```python
from build123d import *

# Parameters (mm, degrees)
SKETCH1_W           = 76.2
SKETCH1_H           = 50.8
SKETCH1_R           = 2.38125
BOSS_EXTRUDE1_DEPTH = 3.0988
FILLET1_R           = 3.175
SKETCH2_W           = 63.5
SKETCH2_H           = 38.1
CUT_EXTRUDE1_DEPTH  = 46.895234627
FILLET3_R           = 3.175


with BuildPart() as part:
    # Sketch1 → Boss-Extrude1 (new body)
    with BuildSketch(Plane.XY):
        Rectangle(SKETCH1_W, SKETCH1_H)
        with Locations((-25.4, 12.7)):
            Circle(SKETCH1_R, mode=Mode.SUBTRACT)
        with Locations((0, 12.7)):
            Circle(SKETCH1_R, mode=Mode.SUBTRACT)
        with Locations((25.4, 12.7)):
            Circle(SKETCH1_R, mode=Mode.SUBTRACT)
        with Locations(Location((25.4, -12.7, 0), (0, 0, 180))):
            Circle(SKETCH1_R, mode=Mode.SUBTRACT)
        with Locations(Location((0, -12.7, 0), (0, 0, 180))):
            Circle(SKETCH1_R, mode=Mode.SUBTRACT)
        with Locations(Location((-25.4, -12.7, 0), (0, 0, 180))):
            Circle(SKETCH1_R, mode=Mode.SUBTRACT)
    extrude(amount=BOSS_EXTRUDE1_DEPTH)

    # Fillet1
    fillet1_edges = [part.edges().sort_by_distance(p)[0] for p in [
        (-38.1, 25.4, 1.5494),
        (38.1, 25.4, 1.5494),
        (38.1, -25.4, 1.5494),
        (-38.1, -25.4, 1.5494),
    ]]
    fillet(fillet1_edges, radius=FILLET1_R)

    # Sketch2 → Cut-Extrude1 (cut, through all)
    with BuildSketch(Plane.XY.offset(3.0988)):
        with BuildLine():
            Line((38.1, -22.225), (38.1, 22.225))
            ThreePointArc((38.1, 22.225), (37.17006403, 24.47006403), (34.925, 25.4))
            Line((34.925, 25.4), (-34.925, 25.4))
            ThreePointArc((-34.925, 25.4), (-37.17006403, 24.47006403), (-38.1, 22.225))
            Line((-38.1, 22.225), (-38.1, -22.225))
            ThreePointArc((-38.1, -22.225), (-37.17006403, -24.47006403), (-34.925, -25.4))
            Line((-34.925, -25.4), (34.925, -25.4))
            ThreePointArc((34.925, -25.4), (37.17006403, -24.47006403), (38.1, -22.225))
        make_face()
        Rectangle(SKETCH2_W, SKETCH2_H, mode=Mode.SUBTRACT)
    extrude(amount=-CUT_EXTRUDE1_DEPTH, mode=Mode.SUBTRACT)

    # Fillet3
    fillet3_edges = [part.edges().sort_by_distance(p)[0] for p in [
        (31.75, -19.05, 1.5494),
        (-31.75, -19.05, 1.5494),
        (-31.75, 19.05, 1.5494),
        (31.75, 19.05, 1.5494),
    ]]
    fillet(fillet3_edges, radius=FILLET3_R)


solid = part.part
```
Check sheet for the modelled part. Datum: model origin and axes. Units: mm. Give positions to 0.01 mm unless a question says otherwise; leave off trailing zeros. Order: outer loops, then holes, each group sorted by start corner. A loop starts at its lowest first (then second) coordinate and runs counter-clockwise, first axis right, second up. Notation, with made-up numbers: M 35,55 L 85,55 A13 ccw 85,72 Z; hole C 58,58 d4. An arc over 180 degrees is marked long. Answer in a Markdown table with one row per item.
1) Gauge pin test, flat end, axial feed: P1, Ø4, axis at x = 0, y = -12.7, coming from the -Z side. Record the tip position at first contact, or that the pin passes through.
Filled sheet:
| item | result |
|---|---|
| P1 | passes through |
2) Release check for a two-part mould opening along Y. For faces 1 (the cylindrical face through (-27.78, 12.8, 1.53)), 2 (the cylindrical face through (30.84, -18.1, 1.53)), 3 (the flat face through (0, 19.05, 2)), 4 (the cylindrical face through (27.78, -12.8, 1.53)) record: +Y half, -Y half, draft (parallel to the pull), parting line (faces both ways), or undercut.
Filled sheet:
| item | result |
|---|---|
| face 1 | undercut |
| face 2 | -Y half |
| face 3 | +Y half |
| face 4 | undercut |
3) Cross-section at D-D, the plane x = 26.5. Enter the section's corners in (y, z), plus the area to 3 significant figures.
Filled sheet:
| item | result |
|---|---|
| outline | M -19.05,0 L -14.81,0 L -14.81,3.1 L -19.05,3.1 Z; M -10.59,0 L 10.59,0 L 10.59,3.1 L -10.59,3.1 Z; M 14.81,0 L 19.05,0 L 19.05,3.1 L 14.81,3.1 Z |
| area | 91.9 mm2 |
4) Cross-section at A-A, the plane x = -25.4. Enter the section's corners in (y, z), plus the area to 3 significant figures.
Filled sheet:
| item | result |
|---|---|
| outline | M -19.05,0 L -15.08,0 L -15.08,3.1 L -19.05,3.1 Z; M -10.32,0 L 10.32,0 L 10.32,3.1 L -10.32,3.1 Z; M 15.08,0 L 19.05,0 L 19.05,3.1 L 15.08,3.1 Z |
| area | 88.5 mm2 |
5) Cross-section at B-B, the plane y = -12.7. Enter the section's corners in (x, z), plus the area to 4 significant figures.
Filled sheet:
| item | result |
|---|---|
| outline | M -31.75,0 L -27.78,0 L -27.78,3.1 L -31.75,3.1 Z; M -23.02,0 L -2.38,0 L -2.38,3.1 L -23.02,3.1 Z; M 2.38,0 L 23.02,0 L 23.02,3.1 L 2.38,3.1 Z; M 27.78,0 L 31.75,0 L 31.75,3.1 L 27.78,3.1 Z |
| area | 152.5 mm2 |
6) Cross-section at C-C, the plane z = 1.05. Count the separate pieces of the cut face and the enclosed holes in it, plus the area to 3 significant figures.
Filled sheet:
| item | result |
|---|---|
| separate pieces | 1 |
| enclosed holes | 6 |
| area | 2,300 mm2 |
7) Thickness scan on L1, parallel to Y at x = 25.4, z = 2.15; L2, parallel to X at y = -12.7, z = 2.1; L3, parallel to X at y = 12, z = 2. Record the ranges inside material, lowest first. Write a range as [from, to].
Filled sheet:
| item | result |
|---|---|
| L1 | y = [-19.05, -15.08], [-10.32, 10.32], [15.08, 19.05] |
| L2 | x = [-31.75, -27.78], [-23.02, -2.38], [2.38, 23.02], [27.78, 31.75] |
| L3 | x = [-31.75, -27.68], [-23.12, -2.28], [2.28, 23.12], [27.68, 31.75] |
